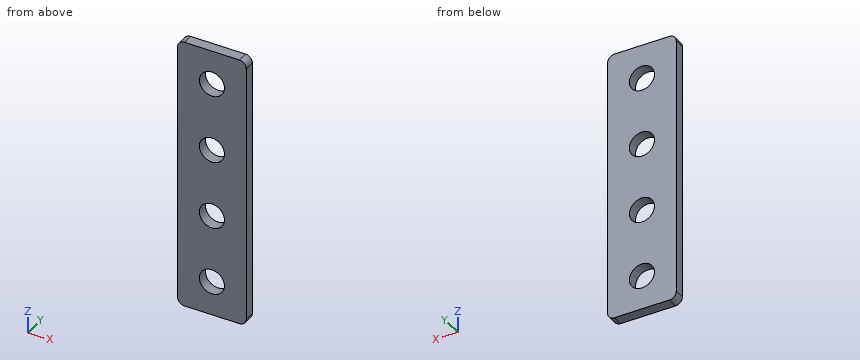
```python
from build123d import *

# Parameters (mm, degrees)
SKETCH1_W           = 10
SKETCH1_H           = 40
SKETCH1_R           = 1.825
BOSS_EXTRUDE1_DEPTH = 1.55
FILLET1_R           = 1


with BuildPart() as part:
    # Sketch1 → Boss-Extrude1 (new body)
    with BuildSketch(Plane(origin=(0, 0, 0), x_dir=(1, 0, 0), z_dir=(0, 1, 0))):
        Rectangle(SKETCH1_W, SKETCH1_H)
        with Locations(Location((0, 15, 0), (0, 0, 90))):
            Circle(SKETCH1_R, mode=Mode.SUBTRACT)
        with Locations(Location((0, 5, 0), (0, 0, 90))):
            Circle(SKETCH1_R, mode=Mode.SUBTRACT)
        with Locations(Location((0, -5, 0), (0, 0, 90))):
            Circle(SKETCH1_R, mode=Mode.SUBTRACT)
        with Locations(Location((0, -15, 0), (0, 0, 90))):
            Circle(SKETCH1_R, mode=Mode.SUBTRACT)
    extrude(amount=BOSS_EXTRUDE1_DEPTH)

    # Fillet1
    fillet1_edges = [part.edges().sort_by_distance(p)[0] for p in [
        (5, 0.775, 20),
        (-5, 0.775, 20),
        (-5, 0.775, -20),
        (5, 0.775, -20),
    ]]
    fillet(fillet1_edges, radius=FILLET1_R)


solid = part.part
```
Geometry check sheet. Reference: the model listing, model coordinates, mm. Give positions to 0.01 mm unless a question says otherwise; leave off trailing zeros. Write each loop counter-clockwise with the first axis right and the second up, starting at its lowest first coordinate (ties: lowest second). Pieces come first, ordered by that corner, then holes.
1) Section check C-C, the plane y = 0.9. Record the boundary of the cut face in (x, z) (3 decimals).
2) Section check A-A, the plane x = 0. Record the boundary of the cut face in (y, z) (3 decimals).
3) Section check B-B, the plane z = -5. Record the boundary of the cut face in (x, y) (3 decimals), and give its area (3 significant figures).
4) Material ranges on L1, parallel to X at y = 1.05, z = -15 (3 decimals); L2, parallel to Z at x = 1, y = 1.15; L3, parallel to Z at x = 0.75, y = 0.65, recorded low to high.
Computed:
1. outline: (-5, -19) arc R1 ccw to (-4, -20) - (4, -20) arc R1 ccw to (5, -19) - (5, 19) arc R1 ccw to (4, 20) - (-4, 20) arc R1 ccw to (-5, 19) - close; hole circle Ø3.65 at (0, -15); hole circle Ø3.65 at (0, -5); hole circle Ø3.65 at (0, 5); hole circle Ø3.65 at (0, 15)
2. outline: (0, -20) - (1.55, -20) - (1.55, -16.825) - (0, -16.825) - close; (0, -13.175) - (1.55, -13.175) - (1.55, -6.825) - (0, -6.825) - close; (0, -3.175) - (1.55, -3.175) - (1.55, 3.175) - (0, 3.175) - close; (0, 6.825) - (1.55, 6.825) - (1.55, 13.175) - (0, 13.175) - close; (0, 16.825) - (1.55, 16.825) - (1.55, 20) - (0, 20) - close
3. outline: (-5, 0) - (-1.825, 0) - (-1.825, 1.55) - (-5, 1.55) - close; (1.825, 0) - (5, 0) - (5, 1.55) - (1.825, 1.55) - close
3. area: 9.84 mm2
4. L1: x = -5 to -1.825, 1.825 to 5
4. L2: z = -20 to -16.53, -13.47 to -6.53, -3.47 to 3.47, 6.53 to 13.47, 16.53 to 20
4. L3: z = -20 to -16.66, -13.34 to -6.66, -3.34 to 3.34, 6.66 to 13.34, 16.66 to 20
